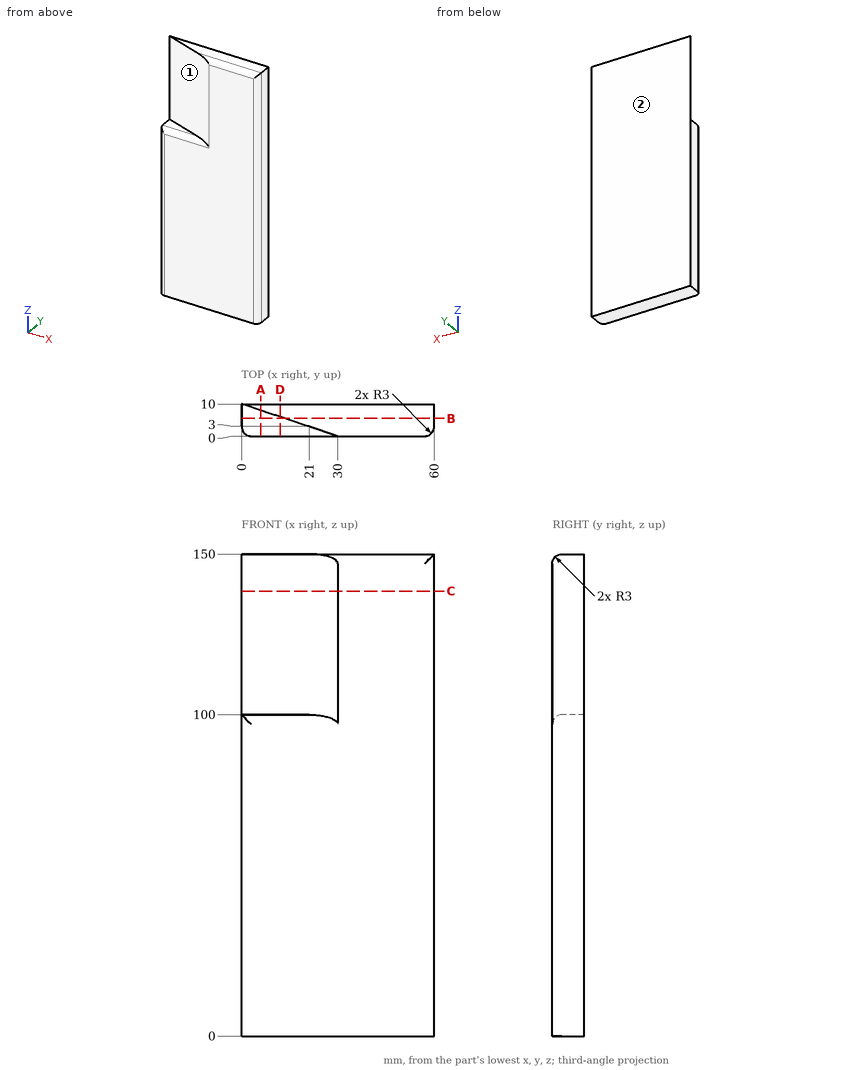
Here's the drawing with two shaded views (mm, measured from the low corner). I have some questions. A direction names the side the tool comes from. Coordinates: 2 decimals unless noted, no trailing zeros. Write each loop counter-clockwise with the first axis right and the second up, starting at its lowest first coordinate (ties: lowest second). Pieces come first, ordered by that corner, then holes. Notation, with made-up numbers: M -3.5,80.5 L 17.5,80.5 A17 cw 17.5,95.5 Z; hole C 11.5,-2.5 d6. An arc over 180 degrees is marked long. Answer as CSV lines item,"result". Start each with the question number.
1) I want a section at A-A, the plane x = 6. Please give me the cut outline in (y, z).
2) I want a section at B-B, the plane y = 5.5. Please give me the cut outline in (x, z), and give its area (4 significant figures).
3) I want a section at C-C, the plane z = 138.5. Please give me the cut outline in (x, y).
4) I want a section at D-D, the plane x = 12. Please give me the cut outline in (y, z), and give its area (3 significant figures).
5) For P1, Ø1.5, axis at x = 11, y = 2.5, coming from the +Z side, with a flat end and sliding along its axis, tell me the tip position at first contact or that it passes through.
6) For the marked faces 1 and 2, which set-ups out of +Z, -Z, +X, -X, +Y, -Y let a thin tool reach every point of the face, with its end or its side?
7) Please list where these lines run through material, in increasing order: line 1 (X direction, y = 2.75, z = 30); line 2 (Z direction, x = 8, y = 7.25); line 3 (Y direction, x = 9, z = 137). Write a range as from..to.
Data:
1,outline,"M 0,0 L 10,0 L 10,150 L 8,150 L 8,100 L 3,100 A3 ccw 0,97 Z"
2,outline,"M 0,0 L 60,0 L 60,150 L 13.5,150 L 13.5,100 L 0,100 Z"
2,area,"8,325 mm^2"
3,outline,"M 0,10 L 30,0 L 57,0 A3 ccw 60,3 L 60,10 Z"
4,outline,"M 0,0 L 10,0 L 10,150 L 6,150 L 6,100 L 3,100 A3 ccw 0,97 Z"
4,area,"1,200 mm^2"
5,P1,"stops at z = 100"
6,face 1,"+Z, -X, -Y"
6,face 2,"+Z, -Z, +X, -X, +Y"
7,line 1,"x = 0.01..59.99"
7,line 2,"z = 0..100"
7,line 3,"y = 7..10"
